```python
from build123d import *

# Parameters (mm, degrees)
SKETCH2_W                        = 114.7
SKETCH2_H                        = 12.5
BRACKETBASE_DEPTH                = 1.75
SKETCH3_R                        = 1.375
BOTTOMCHASSISMOUNTINGHOLES_DEPTH = 1.75
SKETCH4_W                        = 6
SKETCH4_H                        = 16.75
MOUNTINGTABS_DEPTH               = 4.75
SKETCH5_W                        = 6
SKETCH5_H                        = 1.75
EXTENSION_DEPTH                  = 7.75
SKETCH6_R                        = 1.375
REARSHELLMOUNTINGHOLES_DEPTH     = 4.75
SKETCH8_R                        = 3.25
CUT_EXTRUDE2_DEPTH               = 10
SKETCH9_R                        = 3.25
CUT_EXTRUDE3_DEPTH               = 10
SKETCH10_W                       = 6.5
SKETCH10_H                       = 12.5
CUT_EXTRUDE4_DEPTH               = 16
CUT_EXTRUDE4_DEPTH_BACK          = 2.75


with BuildPart() as part:
    # Sketch2 → bracketBase (new body)
    with BuildSketch(Plane(origin=(0, 0, 0), x_dir=(1, 0, 0), z_dir=(0, 1, 0))):
        with Locations((57.35, 6.25)):
            Rectangle(SKETCH2_W, SKETCH2_H)
    extrude(amount=BRACKETBASE_DEPTH)

    # Sketch3 → bottomChassisMountingHoles (cut)
    with BuildSketch(Plane(origin=(0, 1.75, 0), x_dir=(1, 0, 0), z_dir=(0, 1, 0))):
        with Locations((3, 9.75)):
            Circle(SKETCH3_R)
        with Locations((47, 9.75)):
            Circle(SKETCH3_R)
        with Locations((67.7, 9.75)):
            Circle(SKETCH3_R)
        with Locations((111.7, 9.75)):
            Circle(SKETCH3_R)
    extrude(amount=-BOTTOMCHASSISMOUNTINGHOLES_DEPTH, mode=Mode.SUBTRACT)

    # Sketch4 → mountingTabs (add)
    with BuildSketch(Plane.XY):
        with Locations((117.7, 8.375)):
            Rectangle(SKETCH4_W, SKETCH4_H)
        with Locations((-3, 8.375)):
            Rectangle(SKETCH4_W, SKETCH4_H)
        with Locations((57.35, 8.375)):
            Rectangle(SKETCH4_W, SKETCH4_H)
    extrude(amount=-MOUNTINGTABS_DEPTH)

    # Sketch5 → extension (add)
    with BuildSketch(Plane(origin=(0, 0, -12.5), x_dir=(-1, 0, 0), z_dir=(0, 0, -1))):
        with Locations((-117.7, 0.875)):
            Rectangle(SKETCH5_W, SKETCH5_H)
        with Locations((3, 0.875)):
            Rectangle(SKETCH5_W, SKETCH5_H)
    extrude(amount=-EXTENSION_DEPTH)

    # Sketch6 → rearShellMountingHoles (cut)
    with BuildSketch(Plane(origin=(0, 0, -4.75), x_dir=(-1, 0, 0), z_dir=(0, 0, -1))):
        with Locations((-57.35, 12.75)):
            Circle(SKETCH6_R)
        with Locations((-57.35, 5.75)):
            Circle(SKETCH6_R)
        with Locations((-117.7, 12.75)):
            Circle(SKETCH6_R)
        with Locations((-117.7, 5.75)):
            Circle(SKETCH6_R)
        with Locations((3, 5.75)):
            Circle(SKETCH6_R)
        with Locations((3, 12.75)):
            Circle(SKETCH6_R)
    extrude(amount=-REARSHELLMOUNTINGHOLES_DEPTH, mode=Mode.SUBTRACT)

    # Sketch8 → Cut-Extrude2 (cut)
    with BuildSketch(Plane(origin=(0, 1.75, 0), x_dir=(1, 0, 0), z_dir=(0, 1, 0))):
        with Locations((120.95, 8.5675)):
            Circle(SKETCH8_R)
        with Locations((-6.25, 8.5675)):
            Circle(SKETCH8_R)
    extrude(amount=-CUT_EXTRUDE2_DEPTH, mode=Mode.SUBTRACT)

    # Sketch9 → Cut-Extrude3 (cut)
    with BuildSketch(Plane.XZ.offset(-1.75)):
        with Locations((-6.25, -8.5675)):
            Circle(SKETCH9_R)
        with BuildLine():
            Line((120.7, -5.327129651), (122.422971605, -5.194199506))
            Line((122.422971605, -5.194199506), (122.933227388, -11.807870349))
            Line((122.933227388, -11.807870349), (120.7, -11.807870349))
            ThreePointArc((120.7, -11.807870349), (117.7, -8.5675), (120.7, -5.327129651))
        make_face()
    extrude(amount=-CUT_EXTRUDE3_DEPTH, mode=Mode.SUBTRACT)

    # Sketch10 → Cut-Extrude4 (cut, two sides)
    with BuildSketch(Plane(origin=(0, 1.75, 0), x_dir=(1, 0, 0), z_dir=(0, 1, 0))) as cut_extrude4_sk:
        with Locations((117.45, 6.25)):
            Rectangle(SKETCH10_W, SKETCH10_H)
        with Locations((-2.75, 6.25)):
            Rectangle(SKETCH10_W, SKETCH10_H)
    extrude(amount=CUT_EXTRUDE4_DEPTH, mode=Mode.SUBTRACT)
    extrude(cut_extrude4_sk.sketch, amount=-CUT_EXTRUDE4_DEPTH_BACK, mode=Mode.SUBTRACT)


solid = part.part
```
Verification items for the finished model (mm, model axes). A direction names the side the tool comes from. Give positions to 0.01 mm unless a question says otherwise; leave off trailing zeros. Loops run counter-clockwise (first coordinate to the right, second up) from the corner with the lowest first, then second, coordinate; pieces in that order, holes last.
1. Mould release check, pull along Z, two halves, no side actions. Record for faces 4 (the cylindrical face through (2.821, 0.887, -11.113)), 5 (the flat face through (60.35, 9, -2)), 6 (the flat face through (57, 2, 0)): released by +Z, released by -Z, zero draft, split by the parting line, or undercut.
2. Set-up check for faces 1 (the flat face through (57, 9, -4.75)), 2 (the flat face through (54.35, 9, -2)), 3 (the cylindrical face through (69, 0.9, -10.2)): record each of +Z, -Z, +X, -X, +Y, -Y from which the full face is reachable in a straight line by a thin tool's end or side.
3. Section check B-B, the plane y = 12.75. Enter the section's corners in (x, z) (3 decimals), then the cut area to 3 significant figures.
4. Go/stop test with flat-tipped pins: pin 1 Ø4.5 at (x, y) = (57.35, 5.75) entering from +Z; pin 2 Ø4 at (y, z) = (6.5, -3.5) entering from +X; pin 3 Ø3 at (y, z) = (12, -8) entering from +X; pin 4 Ø6 at (x, z) = (39, -6.5) entering from +Y. Record where each tip stops, or that it passes through.
5. Thickness scan on line 1 (X direction, y = 1.45, z = -9.75) (3 decimals); line 2 (Z direction, x = 3, y = 1.3) (3 decimals); line 3 (Z direction, x = 55.5, y = 3.75). Record the ranges inside material, lowest first.
6. Section check C-C, the plane z = -2.25. Enter the section's corners in (x, y) (3 decimals), then the cut area to 3 significant figures.
7. Section check D-D, the plane x = 57.35. Enter the section's corners in (y, z) (3 decimals).
8. Section check A-A, the plane x = 3. Enter the section's corners in (y, z) (3 decimals).
Geometry says:
1. face 4: undercut
1. face 5: zero draft
1. face 6: released by +Z
2. face 1: -Z, +X, -X, +Y
2. face 2: +Z, -Z, -X, +Y
2. face 3: +Y, -Y
3. outline: (54.35, -4.75) - (55.975, -4.75) - (55.975, 0) - (54.35, 0) - close; (58.725, -4.75) - (60.35, -4.75) - (60.35, 0) - (58.725, 0) - close
3. area: 15.4 mm2
4. pin 1: stops at z = 0
4. pin 2: stops at x = 60.35
4. pin 3: passes through
4. pin 4: stops at y = 1.75
5. line 1: x = 0.5 to 1.625, 4.375 to 45.625, 48.375 to 66.325, 69.075 to 110.325, 113.075 to 114.2
5. line 2: z = -12.5 to -11.125, -8.375 to 0
5. line 3: z = -4.75 to 0
6. outline: (0.5, 0) - (114.2, 0) - (114.2, 1.75) - (60.35, 1.75) - (60.35, 16.75) - (54.35, 16.75) - (54.35, 1.75) - (0.5, 1.75) - close; hole circle Ø2.75 at (57.35, 5.75); hole circle Ø2.75 at (57.35, 12.75)
6. area: 277 mm2
7. outline: (0, -12.5) - (1.75, -12.5) - (1.75, -4.75) - (4.375, -4.75) - (4.375, 0) - (0, 0) - close; (7.125, -4.75) - (11.375, -4.75) - (11.375, 0) - (7.125, 0) - close; (14.125, -4.75) - (16.75, -4.75) - (16.75, 0) - (14.125, 0) - close
8. outline: (0, -12.5) - (1.75, -12.5) - (1.75, -11.125) - (0, -11.125) - close; (0, -8.375) - (1.75, -8.375) - (1.75, 0) - (0, 0) - close
